from build123d import *

# Parameters (mm, degrees)
FURO_ROSCADO_DE_M181_D                     = 15.5
FURO_ROSCADO_DE_M181_DEPTH                 = 25
FURO_ROSCADO_DE_M181_CSINK_D               = 18.05
FURO_ROSCADO_DE_M181_CSINK_ANGLE           = 90
FURO_ROSCADO_DE_M181_TIP                   = 4.656669797
FURO_ROSCADO_DE_M181_ON_FACE_2_D           = 15.5
FURO_ROSCADO_DE_M181_ON_FACE_2_DEPTH       = 25
FURO_ROSCADO_DE_M181_ON_FACE_2_CSINK_D     = 18.05
FURO_ROSCADO_DE_M181_ON_FACE_2_CSINK_ANGLE = 90
FURO_ROSCADO_DE_M181_ON_FACE_2_TIP         = 4.656669797


with BuildPart() as part:
    # Esboço1 → Revolução1 (revolve)
    with BuildSketch(Plane.XY):
        Polygon((0, 0), (0, 18), (50, 18), (50, 22), (100, 22), (100, 20), (525, 20), (525, 18), (575, 18), (575, 0), align=None)
    revolve(axis=Axis((575, 0, 0), (-1, 0, 0)))

    # Furo roscado de M181
    with Locations(Plane(origin=(0, 0, 0), x_dir=(0, -1, 0), z_dir=(-1, 0, 0))):
        with Locations((0, 0)):
            CounterSinkHole(FURO_ROSCADO_DE_M181_D / 2, FURO_ROSCADO_DE_M181_CSINK_D / 2, depth=FURO_ROSCADO_DE_M181_DEPTH, counter_sink_angle=FURO_ROSCADO_DE_M181_CSINK_ANGLE)
            with Locations((0, 0, -(FURO_ROSCADO_DE_M181_DEPTH + FURO_ROSCADO_DE_M181_TIP / 2))):  # 118° drill point
                Cone(0, FURO_ROSCADO_DE_M181_D / 2, FURO_ROSCADO_DE_M181_TIP, mode=Mode.SUBTRACT)

    # Furo roscado de M181 on face 2
    with Locations(Plane(origin=(575, 0, 0), x_dir=(0, 0, 1), z_dir=(1, 0, 0))):
        with Locations((0, 0)):
            CounterSinkHole(FURO_ROSCADO_DE_M181_ON_FACE_2_D / 2, FURO_ROSCADO_DE_M181_ON_FACE_2_CSINK_D / 2, depth=FURO_ROSCADO_DE_M181_ON_FACE_2_DEPTH, counter_sink_angle=FURO_ROSCADO_DE_M181_ON_FACE_2_CSINK_ANGLE)
            with Locations((0, 0, -(FURO_ROSCADO_DE_M181_ON_FACE_2_DEPTH + FURO_ROSCADO_DE_M181_ON_FACE_2_TIP / 2))):  # 118° drill point
                Cone(0, FURO_ROSCADO_DE_M181_ON_FACE_2_D / 2, FURO_ROSCADO_DE_M181_ON_FACE_2_TIP, mode=Mode.SUBTRACT)


solid = part.part
For this review, take the finished solid that the model builds, in its own axes (mm). A direction names the side the tool comes from. Give positions to 0.01 mm unless a question says otherwise; leave off trailing zeros. Loops run counter-clockwise (first coordinate to the right, second up) from the corner with the lowest first, then second, coordinate; pieces in that order, holes last. Notation, with made-up numbers: M 61,20.5 L 92,20.5 A18 ccw 92,25.5 Z; hole C 46,27 d2. An arc over 180 degrees is marked long. Answer as a JSON object with one key per item and string values. Group by question number.
Q1. Add section B-B on x = 231. Give the boundary of the cut face in (y, z).
Q2. For probe 1 along Y at (x, z) = (13.5, 0); probe 2 along X at (y, z) = (18, 3.5), list the stretches that pass through material, from the lowest coordinate up. Write a range as [from, to].
Q3. Add section A-A on x = 41.5. Give the boundary of the cut face in (y, z), and give its area (3 significant figures).
Q4. Insertion check: P1, Ø2, axis at y = 9.5, z = 17, coming from the -X side; P2, Ø8, axis at x = 125.5, z = -1.5, coming from the +Y side; P3, Ø4, axis at y = -3.5, z = 0.5, coming from the -X side. Each pin has a flat end and moves straight along its axis. Give the tip position at first contact, or say it passes through.
Q5. Tool access review of faces 1 (the flat face through (575, -8.3, -4.3)), 2 (the cylindrical face through (561.696, -7.684, 1.009)), 3 (the cylindrical face through (25.35, -2.343, -17.847)): name each direction out of +Z, -Z, +X, -X, +Y, -Y from which nothing blocks a thin tool from reaching the whole face with its end or side.
Q6. Mouldability with a two-part tool opening along Y and no side actions: class faces 4 (the cylindrical face through (13.304, -1.009, 7.684)), 5 (the conical face through (28.85, 0.29, -1.31)), 6 (the flat face through (50, 8.3, 16.2)), 7 (the cylindrical face through (75.35, -4.769, 21.477)) as +Y half, -Y half, draft (parallel to the pull), parting line (faces both ways), or undercut.
Checked values:
{
 "1": {"outline": "C 0,0 d40"},
 "2": {"probe 1": "[-18, -7.75], [7.75, 18]", "probe 2": "[50, 525]"},
 "3": {"outline": "C 0,0 d36", "area": "1,020 mm²"},
 "4": {"P1": "x = 50", "P2": "y = 20", "P3": "x = 26.33"},
 "5": {"face 1": "+Z, -Z, +X, +Y, -Y", "face 2": "+X", "face 3": "-X"},
 "6": {"face 4": "undercut", "face 5": "undercut", "face 6": "draft", "face 7": "parting line"}
}
